Verification items for the finished model (mm, model axes). Give positions to 0.01 mm unless a question says otherwise; leave off trailing zeros. Order: outer loops, then holes, each group sorted by start corner. A loop starts at its lowest first (then second) coordinate and runs counter-clockwise, first axis right, second up. Notation, with made-up numbers: (51, 24.25) - (59, 24.25) arc R24 ccw to (59, 57.25) - close; hole circle Ø3 at (30.5, -11.5). An arc over 180 degrees is marked (long way). Answer as a JSON object with one key per item and string values.
Autodesk Inventor part; units mm, degrees
ref_plane "YZ Plane" through (0, 0, 0) normal (1, 0, 0) x (0, 1, 0)
ref_plane "XZ Plane" through (0, 0, 0) normal (0, 1, 0) x (-1, 0, 0)
ref_plane "XY Plane" through (0, 0, 0) normal (0, 0, 1) x (1, 0, 0)
sketch "Sketch1" plane through (0, 0, 0) normal (0, 0, 1) x (1, 0, 0)
  line L0 (-12.7, -12.7) -> (12.7, -12.7)
  line L1 (12.7, -12.7) -> (12.7, 12.7)
  line L2 (12.7, 12.7) -> (-12.7, 12.7)
  line L3 (-12.7, 12.7) -> (-12.7, -12.7)
  line L4 (-12.7, -12.7) -> (12.7, 12.7) construction
  line L5 (12.7, -12.7) -> (-12.7, 12.7) construction
  point P0 (0, 0)
  dimension "d0" = 25.4
  dimension "d1" = 25.4
extrude "Extrusion1" add sketch "Sketch1" along normal blind 88.9
sketch "Sketch2" plane through (12.7, -12.7, 0) normal (1, 0, 0) x (0, 0, -1)
  line L0 (-88.9, 0) -> (-88.9, 25.4)
  line L1 (0, 0) -> (0, 25.4)
  line L2 (0, 0) -> (-88.9, 0)
  point P0 (0, 12.7)
  point P1 (-69.85, 12.7)
  point P2 (-19.05, 12.7)
  dimension "d4" = 19.05
  dimension "d5" = 88.9
  dimension "d7" = 19.05
  dimension "d27" = 25.4
  dimension "d28" = 12.7
hole "Hole1" at (12.7, 0, 69.85) at (12.7, 0, 19.05) direction (-1, 0, 0) diameter 3.9624 depth 12.7 tip angle 118
sketch "Sketch3" plane through (-12.7, 12.7, 0) normal (0, 1, 0) x (1, 0, 0)
  line L0 (12.7, -21.0312) -> (12.7, -17.0688)
  line L1 (12.7, -71.8312) -> (12.7, -67.8688)
  line L2 (25.4, -88.9) -> (0, -88.9)
  line L3 (25.4, 0) -> (0, 0)
  line L4 (0, 0) -> (0, -88.9)
  point P0 (12.7, 0)
  point P1 (12.7, -19.05)
  point P2 (12.7, -69.85)
hole "Hole2" at (0, 12.7, 19.05) at (0, 12.7, 69.85) direction (0, -1, 0) diameter 3.9624 depth 12.7 tip angle 118
sketch "Sketch4" plane through (0, 0, 88.9) normal (0, 0, 1) x (1, 0, 0)
  point P0 (0, 0)
  point P1 (0, 0)
hole "Hole3" at (0, 0, 88.9) direction (0, 0, -1) diameter 3.9624 depth 25.4 tip angle 118
sketch "Sketch5" plane through (0, 0, 0) normal (0, 0, -1) x (-1, 0, 0)
  point P0 (0, 0)
  point P1 (0, 0)
hole "Hole4" at (0, 0, 0) direction (0, 0, 1) diameter 3.9624 depth 25.4 tip angle 118
properties part number "CH3-DiffBoxGussetBlock"
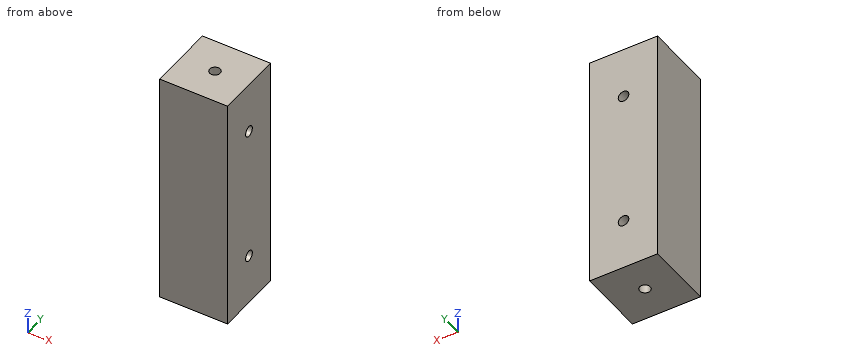
(1) Section check A-A (z = 19.05). Record the cut outline in (x, y).
Computed values:
{"outline": "(-12.7, -12.7) - (12.7, -12.7) - (12.7, -1.98) - (0, -1.98) arc R1.98 cw to (-1.98, 0) - (-1.98, 12.7) - (-12.7, 12.7) - close; (1.98, 1.98) - (12.7, 1.98) - (12.7, 12.7) - (1.98, 12.7) - close"}
(2) Gauge pin test, flat end, axial feed: pin 1 Ø3.5 at (y, z) = (0, 19.05) entering from +X. Record the tip position at first contact, or that the pin passes through.
Computed values:
{"pin 1": "stops at x = -0.93"}
(3) Material ranges on line 1 along Z through (x, y) = (0, 3.75); line 2 along Y through (x, z) = (0, 9.75); line 3 along Z through (x, y) = (4, 1.5), recorded low to high. Write a range as [from, to].
Computed values:
{"line 1": "z = [0, 17.07], [21.03, 67.87], [71.83, 88.9]", "line 2": "y = [-12.7, -1.98], [1.98, 12.7]", "line 3": "z = [0, 17.76], [20.34, 68.56], [71.14, 88.9]"}
(4) Section check B-B (z = 6). Record the cut outline in (x, y), then the cut area to 3 significant figures.
Computed values:
{"outline": "(-12.7, -12.7) - (12.7, -12.7) - (12.7, 12.7) - (-12.7, 12.7) - close; hole circle Ø3.96 at (0, 0)", "area": "633 mm²"}
